```python
from build123d import *

# Parameters (mm, degrees)
F0_W      = 20
F0_H      = 200
F1_DEPTH  = 688
F2_W      = 18.5
F2_H      = 160
F3_DEPTH  = 688
F4_W      = 17
F4_H      = 38.5
F5_DEPTH  = 688
F6_W      = 100
F6_H      = 200
F7_DEPTH  = 1.5
F8_W      = 17
F8_H      = 40
F9_DEPTH  = 80
F10_W     = 15.5
F10_H     = 38.5
F11_DEPTH = 78.5


with BuildPart() as f1:
    # F0 (on Front) → F1 (new body)
    with BuildSketch(Plane.XZ):
        Rectangle(F0_W, F0_H)
    extrude(amount=F1_DEPTH)

    # F2 (on face) → F3 (cut)
    with BuildSketch(Plane.XZ.offset(688)):
        with Locations((0.75, -20)):
            Rectangle(F2_W, F2_H)
    extrude(amount=-F3_DEPTH, mode=Mode.SUBTRACT)

    # F4 (on face) → F5 (cut)
    with BuildSketch(Plane.XZ.offset(688)):
        with Locations((0, 79.25)):
            Rectangle(F4_W, F4_H)
    extrude(amount=-F5_DEPTH, mode=Mode.SUBTRACT)

    # F6 (on face) → F7 (join)
    with BuildSketch(Plane.XZ.offset(688)):
        with Locations((40, 0)):
            Rectangle(F6_W, F6_H)
    extrude(amount=F7_DEPTH)

    # F8 (on face) → F9 (join)
    with BuildSketch(Plane.YZ.offset(10)):
        with Locations((-679.5, 80)):
            Rectangle(F8_W, F8_H)
    extrude(amount=F9_DEPTH)

    # F10 (on face) → F11 (cut)
    with BuildSketch(Plane.YZ.offset(90)):
        with Locations((-680.25, 79.25)):
            Rectangle(F10_W, F10_H)
    extrude(amount=-F11_DEPTH, mode=Mode.SUBTRACT)


solid = f1.part
```
The listing builds one solid part. Answer for the finished solid, in the listing's coordinates (mm). A direction names the side the tool comes from. Round coordinates to 2 decimals unless told otherwise and drop trailing zeros. Loops run counter-clockwise (first coordinate to the right, second up) from the corner with the lowest first, then second, coordinate; pieces in that order, holes last.
Q1. For a pull along X with two mould halves and no side action, classify faces 6 (the face through (-10, -340, -1)), 7 (the face through (8.5, -349, 79)), 8 (the face through (9.8, -345.6, 60)), 9 (the face through (0, -349, 98.5)) as released by +X, released by -X, zero draft, split by the parting line, or undercut.
Q2. Section D-D, the plane x = -2 is taken. Determine the outline of the cut face in (y, z), then the cut area to 3 significant figures.
Q3. Which of the six approach directions +Z, -Z, +X, -X, +Y, -Y give full straight-line access (tool end or side, diameter ignored) to faces 1 (the face through (10, -331, 80)), 2 (the face through (90, -689, 15)), 3 (the face through (-8.5, -349, -2)), 4 (the face through (51, -672.5, 79)), 5 (the face through (-9, 0, 15))?
Q4. Given pin 1 Ø20 at (x, z) = (39, 77) entering from +Y; pin 2 Ø6 at (y, z) = (-260.5, 0.5) entering from +X; pin 3 Ø13.5 at (x, y) = (4, -354.5) entering from -Z, each flat-ended and moving along its own axis, determine where each tip first touches the part or whether it passes through.
Q5. Find the intervals of material crossed by line 1 (X direction, y = -470, z = 74); line 2 (Y direction, x = 71, z = 62); line 3 (Y direction, x = 43, z = -51.5), in increasing order.
Q6. Section A-A, the plane y = -346 is taken. Determine the outline of the cut face in (x, z).
Q7. Section B-B, the plane x = 32.5 is taken. Determine the outline of the cut face in (y, z).
Q8. Section C-C, the plane z = -84 is taken. Determine the outline of the cut face in (x, y).
Completed:
1. face 6: released by -X
1. face 7: undercut
1. face 8: zero draft
1. face 9: undercut
2. outline: (-689.5, -100) - (-688, -100) - (-688, 98.5) - (0, 98.5) - (0, 100) - (-689.5, 100) - close
2. area: 1,330 mm2
3. face 1: +Z, -Z, +X, +Y
3. face 2: +Z, -Z, +X, +Y, -Y
3. face 3: -Z, +Y
3. face 4: -Z, +X
3. face 5: +Z, -Z, +X, -X, +Y
4. pin 1: stops at y = -671
4. pin 2: stops at x = -8.5
4. pin 3: stops at z = 60
5. line 1: x = -10 to -8.5, 8.5 to 10
5. line 2: y = -689.5 to -688, -672.5 to -671
5. line 3: y = -689.5 to -688
6. outline: (-10, -100) - (-8.5, -100) - (-8.5, 98.5) - (8.5, 98.5) - (8.5, 60) - (10, 60) - (10, 100) - (-10, 100) - close
7. outline: (-689.5, -100) - (-688, -100) - (-688, 98.5) - (-672.5, 98.5) - (-672.5, 60) - (-671, 60) - (-671, 100) - (-689.5, 100) - close
8. outline: (-10, -689.5) - (90, -689.5) - (90, -688) - (-8.5, -688) - (-8.5, 0) - (-10, 0) - close
